Check sheet for the modelled part. Datum: model origin and axes. Units: mm. A direction names the side the tool comes from. Give positions to 0.01 mm unless a question says otherwise; leave off trailing zeros. Loops run counter-clockwise (first coordinate to the right, second up) from the corner with the lowest first, then second, coordinate; pieces in that order, holes last. Notation, with made-up numbers: M -24,40 L -8,40 A24 cw -8,54 Z; hole C 22.25,2.5 d8. An arc over 180 degrees is marked long. Write each question's results on one line, items separated by ' | '. Start each with the question number.
1. Go/stop test with flat-tipped pins: pin 1 (4 mm diameter, centred on y = -4, z = 7, fed in from +X); pin 2 (7.5 mm diameter, centred on x = 56.5, y = -18, fed in from +Z); pin 3 (8 mm diameter, centred on x = -4.5, z = 52, fed in from +Y); pin 4 (12.5 mm diameter, centred on x = 57, y = -17.5, fed in from -Z). Record where each tip stops, or that it passes through.
2. Tool access check on faces 4 (the flat face through (4, -12.7, 2)), 5 (the flat face through (56, -4, 52.098)), 6 (the flat face through (-39.499, -6, 0)), 7 (the flat face through (49.401, -6, 1)), 8 (the flat face through (56, -4, -49.502)). Record the directions out of +Z, -Z, +X, -X, +Y, -Y that give a thin tool (end or side, any length) a straight path to the whole face; none if there is none.
3. Sectioned sample at C-C on x = 38.5. Record the cut outline in (y, z).
4. Material ranges on line 1 along Z through (x, y) = (54, -1.5); line 2 along X through (y, z) = (-2.75, 0.5); line 3 along Y through (x, z) = (36, -35), recorded low to high.
5. Sectioned sample at A-A on z = 18. Record the cut outline in (x, y) (3 decimals).
6. Draft check along X on faces 1 (the cylindrical face through (52.585, -12.281, -30.186)), 2 (the flat face through (11, 0, 2)), 3 (the flat face through (49.401, -6, 65)). Enter one of: pulls with the +X half, pulls with the -X half, needs draft (parallel to the pull), parting line crosses it, or undercut.
7. Sectioned sample at B-B on z = 68. Record the cut outline in (x, y).
```python
from build123d import *

# Parameters (mm, degrees)
F0_W     = 101.6
F0_H     = 152.4
F1_DEPTH = 12.7
F3_DEPTH = 152.4
F4_R     = 9.525
F5_DEPTH = 152.4
F7_W     = 50.8
F7_H     = 25.4
F8_DEPTH = 50.8


# Not quite as in the source:
# - a feature names something its author has since deleted; it is built from what else it names


with BuildPart() as f1:
    # F0 (on Front) → F1 (new body)
    with BuildSketch(Plane.XZ):
        with Locations((11.3006858155, 1.2977712616)):
            Rectangle(F0_W, F0_H)
    extrude(amount=F1_DEPTH)

    # F2 (on face) → F3 (join)
    with BuildSketch(Plane.XY.offset(77.4977712616)):
        with BuildLine():
            ThreePointArc((49.4006858155, -12.7), (62.1006858155, -25.4), (74.8006858155, -12.7))
            ThreePointArc((74.8006858155, -12.7), (71.0809419366, -3.7197438789), (62.1006858155, 0))
            Line((62.1006858155, 0), (62.1006858155, -12.7))
            Line((62.1006858155, -12.7), (49.4006858155, -12.7))
        make_face()
    extrude(amount=-F3_DEPTH)

    # F4 (on face) → F5 (cut, through all)
    with BuildSketch(Plane.XY.offset(77.4977712616)):
        with Locations((62.1006858155, -12.7)):
            Circle(F4_R)
    extrude(amount=-F5_DEPTH, mode=Mode.SUBTRACT)

    # F7 (on offset) → F8 (cut)
    with BuildSketch(Plane.XZ.offset(25.4)):
        with Locations((74.8006858155, 64.7977712616)):
            Rectangle(F7_W, F7_H)
        with Locations((74.8006858155, -62.2022287384)):
            Rectangle(F7_W, F7_H)
        with Locations((74.8006858155, 1.2977712616)):
            Rectangle(F7_W, F7_H)
    extrude(amount=-F8_DEPTH, mode=Mode.SUBTRACT)


solid = f1.part
```
Output values:
1) pin 1: x = 49.4 | pin 2: z = 52.1 | pin 3: y = 0 | pin 4: z = -49.5
2) face 4: +Z, -Z, -X, -Y | face 5: +Z, +X, +Y, -Y | face 6: +Z, -Z, -X, +Y, -Y | face 7: +X, +Y, -Y | face 8: -Z, +X, +Y, -Y
3) outline: M -12.7,-74.9 L 0,-74.9 L 0,77.5 L -12.7,77.5 Z
4) line 1: -49.5 to -11.4, 14 to 52.1 | line 2: -39.5 to 49.4 | line 3: -12.7 to 0
5) outline: M -39.499,-12.7 L 49.401,-12.7 A12.7 ccw long 62.101,0 L -39.499,0 Z; hole C 62.101,-12.7 d19.05
6) face 1: undercut | face 2: needs draft | face 3: pulls with the +X half
7) outline: M -39.5,-12.7 L 49.4,-12.7 L 49.4,0 L -39.5,0 Z
